Design review of the part built by this model. Coordinates are the model's own, in mm. Face numbers are marked on the shaded views. A direction names the side the tool comes from. Coordinates: 2 decimals unless noted, no trailing zeros. Write each loop counter-clockwise with the first axis right and the second up, starting at its lowest first coordinate (ties: lowest second). Pieces come first, ordered by that corner, then holes.
Q1. For probe 1 along Y at (x, z) = (0, -10.7) (3 decimals); probe 2 along Y at (x, z) = (-10.6, 0) (3 decimals); probe 3 along Z at (x, y) = (10.5, 50.8) (3 decimals), list the stretches that pass through material, from the lowest coordinate up.
Q2. Machinability: for the marked faces 5 and 6, which of the approach directions +Z, -Z, +X, -X, +Y, -Y give a long, thin tool a straight path to every point of the face, cutting with its end or side? Answer none if there is none.
Q3. Mouldability with a two-part tool opening along X and no side actions: class the marked faces 1, 2, 3 and 4 as pulls with the +X half, pulls with the -X half, needs draft (parallel to the pull), parting line crosses it, or undercut.
Q4. Take a section at B-B (z = 8.25). Give the boundary of the cut face in (x, y) (3 decimals), and give its area (3 significant figures).
Q5. Take a section at D-D (z = 0). Give the boundary of the cut face in (x, y) (3 decimals).
Q6. Take a section at C-C (x = -4.5). Give the boundary of the cut face in (y, z) (3 decimals), and give its area (3 significant figures).
Q7. Take a section at A-A (y = 12.7). Give the boundary of the cut face in (x, z) (3 decimals).
Autodesk Inventor part; units mm, degrees
ref_plane "YZ Plane" through (0, 0, 0) normal (1, 0, 0) x (0, 1, 0)
ref_plane "XZ Plane" through (0, 0, 0) normal (0, 1, 0) x (-1, 0, 0)
ref_plane "XY Plane" through (0, 0, 0) normal (0, 0, 1) x (1, 0, 0)
sketch "Sketch1" plane through (0, 0, 0) normal (0, 1, 0) x (-1, 0, 0)
  line L0 (-12.7, -12.7) -> (12.7, -12.7)
  line L1 (12.7, -12.7) -> (12.7, 12.7)
  line L2 (12.7, 12.7) -> (-12.7, 12.7)
  line L3 (-12.7, 12.7) -> (-12.7, -12.7)
  line L4 (-12.7, -12.7) -> (12.7, 12.7) construction
  line L5 (12.7, -12.7) -> (-12.7, 12.7) construction
  line L6 (-9.525, -9.525) -> (9.525, -9.525)
  line L7 (9.525, -9.525) -> (9.525, 9.525)
  line L8 (9.525, 9.525) -> (-9.525, 9.525)
  line L9 (-9.525, 9.525) -> (-9.525, -9.525)
  line L10 (-9.525, -9.525) -> (9.525, 9.525) construction
  line L11 (9.525, -9.525) -> (-9.525, 9.525) construction
  point P0 (0, 0)
  dimension "d0" = 25.4
  dimension "d1" = 25.4
  dimension "d2" = 19.05
  dimension "d3" = 19.05
extrude "Extrusion1" add sketch "Sketch1" along normal blind 152.4
sketch "Sketch2" plane through (-12.7, 0, 12.7) normal (0, 0, 1) x (1, 0, 0)
  line L0 (0, 152.4) -> (25.4, 152.4)
  line L1 (0, 0) -> (0, 152.4)
  line L2 (12.7, 152.4) -> (12.7, 139.7)
  line L3 (12.7, 139.7) -> (12.7, 101.6)
  circle A0 centre (12.7, 139.7) radius 3.175
  circle A1 centre (12.7, 101.6) radius 3.175
  point P0 (12.7, 0)
  dimension "d6" = 12.7
  dimension "d7" = 38.1
  dimension "d8" = 180
  dimension "d9" = 6.35
  dimension "d10" = 6.35
extrude "Extrusion2" cut sketch "Sketch2" against normal blind 25.4
sketch "Sketch3" plane through (12.7, 0, 12.7) normal (1, 0, 0) x (0, 0, -1)
  line L0 (0, 0) -> (0, 152.4)
  line L1 (12.7, 0) -> (12.7, 12.7)
  line L2 (12.7, 0) -> (25.4, 0) construction
  line L3 (12.7, 12.7) -> (12.7, 50.8)
  line L4 (12.7, 12.7) -> (50.8, 12.7) construction
  circle A0 centre (12.7, 50.8) radius 3.175
  circle A1 centre (12.7, 12.7) radius 3.175
  dimension "d13" = 12.7
  dimension "d14" = 90
  dimension "d15" = 38.1
  dimension "d16" = 90
  dimension "d17" = 6.35
  dimension "d18" = 6.35
extrude "Extrusion3" cut sketch "Sketch3" against normal blind 25.4
properties part number "SuperStructureSupport"
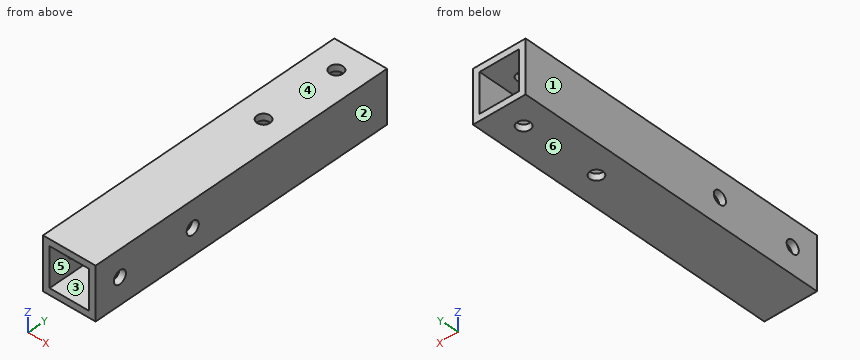
Response:
1. probe 1: y = 0 to 98.425, 104.775 to 136.525, 142.875 to 152.4
1. probe 2: y = 0 to 9.525, 15.875 to 47.625, 53.975 to 152.4
1. probe 3: z = -12.7 to -3.175, 3.175 to 12.7
2. face 5: +Y, -Y
2. face 6: -Z, +X, -X, +Y, -Y
3. face 1: pulls with the -X half
3. face 2: pulls with the +X half
3. face 3: undercut
3. face 4: needs draft
4. outline: (-12.7, 0) - (-9.525, 0) - (-9.525, 152.4) - (-12.7, 152.4) - close; (9.525, 0) - (12.7, 0) - (12.7, 152.4) - (9.525, 152.4) - close
4. area: 968 mm2
5. outline: (-12.7, 0) - (-9.525, 0) - (-9.525, 9.525) - (-12.7, 9.525) - close; (-12.7, 15.875) - (-9.525, 15.875) - (-9.525, 47.625) - (-12.7, 47.625) - close; (-12.7, 53.975) - (-9.525, 53.975) - (-9.525, 152.4) - (-12.7, 152.4) - close; (9.525, 0) - (12.7, 0) - (12.7, 9.525) - (9.525, 9.525) - close; (9.525, 15.875) - (12.7, 15.875) - (12.7, 47.625) - (9.525, 47.625) - close; (9.525, 53.975) - (12.7, 53.975) - (12.7, 152.4) - (9.525, 152.4) - close
6. outline: (0, -12.7) - (152.4, -12.7) - (152.4, -9.525) - (0, -9.525) - close; (0, 9.525) - (152.4, 9.525) - (152.4, 12.7) - (0, 12.7) - close
6. area: 968 mm2
7. outline: (-12.7, -12.7) - (12.7, -12.7) - (12.7, -3.175) - (9.525, -3.175) - (9.525, -9.525) - (-9.525, -9.525) - (-9.525, -3.175) - (-12.7, -3.175) - close; (-12.7, 3.175) - (-9.525, 3.175) - (-9.525, 9.525) - (9.525, 9.525) - (9.525, 3.175) - (12.7, 3.175) - (12.7, 12.7) - (-12.7, 12.7) - close
